```python
from build123d import *

# Parameters (mm, degrees)
F0_W     = 80
F0_H     = 40
F1_DEPTH = 5
F2_W     = 30
F2_H     = 5.5
F3_DEPTH = 20
F4_W     = 40
F4_H     = 7
F5_DEPTH = 22.4


with BuildPart() as f1:
    # F0 (on Top) → F1 (new body)
    with BuildSketch(Plane.XY):
        Rectangle(F0_W, F0_H)
    extrude(amount=F1_DEPTH)

    # F2 (on face) → F3 (join)
    with BuildSketch(Plane.XY.offset(5)):
        with Locations((-25, -17.25)):
            Rectangle(F2_W, F2_H)
        with Locations((-25, 17.25)):
            Rectangle(F2_W, F2_H)
    extrude(amount=F3_DEPTH)

    # F4 (on face) → F5 (cut)
    with BuildSketch(Plane.XY.offset(5)):
        with Locations((15, 0)):
            Rectangle(F4_W, F4_H)
    extrude(amount=-F5_DEPTH, mode=Mode.SUBTRACT)


solid = f1.part
```
The listing builds one solid part. Answer for the finished solid, in the listing's coordinates (mm). A direction names the side the tool comes from. Give positions to 0.01 mm unless a question says otherwise; leave off trailing zeros. Order: outer loops, then holes, each group sorted by start corner. A loop starts at its lowest first (then second) coordinate and runs counter-clockwise, first axis right, second up. Notation, with made-up numbers: (-39, 62) -> (18, 62) arc R27 ccw to (18, 97) -> close; hole circle Ø10 at (42.25, 34). An arc over 180 degrees is marked (long way). Answer as a JSON object with one key per item and string values. Group by question number.
Item 1: The part is cut by section D-D on x = -14.5. Write down the section's boundary in (y, z).
Item 2: Consider L1, parallel to Y at x = -30.5, z = 13.75; L2, parallel to X at y = 18, z = 5.5; L3, parallel to Z at x = 21, y = 11. Determine where each line is inside the solid, lowest interval first. Write a range as from..to.
Item 3: Flat-ended cylindrical pins translate along their axes: pin 1 (10 mm diameter, centred on x = -13, y = -12, fed in from +Z); pin 2 (20 mm diameter, centred on x = -18, y = 0, fed in from +Z); pin 3 (6 mm diameter, centred on y = 12, z = 14, fed in from +X); pin 4 (2 mm diameter, centred on x = -1, y = -1.5, fed in from -Z). Find the tip coordinate at first contact, or state that the pin passes through.
Item 4: A tool of negligible diameter and unlimited length cuts with its end or side. For faces 1 (the flat face through (15, -3.5, 3)), 2 (the flat face through (-10, 17, 15)), 3 (the flat face through (-25, 14.5, 15)), 4 (the flat face through (-25, -17, 25)), from which of +Z, -Z, +X, -X, +Y, -Y can it reach the whole face along a straight path? Write none if from no direction.
Item 5: The part is cut by section A-A on x = 4.5. Write down the section's boundary in (y, z).
Item 6: The part is cut by section C-C on z = 2.75. Write down the section's boundary in (x, y).
Item 7: The part is cut by section B-B on z = 10.5. Write down the section's boundary in (x, y).
Item 8: Determine the mould class of faces 5 (the flat face through (-40, 0, 4)), 6 (the flat face through (15, 3.5, 3)), 7 (the flat face through (-10, -17, 15)), 8 (the flat face through (-1, 5, 5)) for opening direction X: pulls with the +X half, pulls with the -X half, needs draft (parallel to the pull), parting line crosses it, or undercut.
Result set:
{
 "1": {"outline": "(-20, 0) -> (20, 0) -> (20, 25) -> (14.5, 25) -> (14.5, 5) -> (-14.5, 5) -> (-14.5, 25) -> (-20, 25) -> close"},
 "2": {"L1": "-20..-14.5, 14.5..20", "L2": "-40..-10", "L3": "0..5"},
 "3": {"pin 1": "z = 25", "pin 2": "z = 5", "pin 3": "x = -10", "pin 4": "through"},
 "4": {"face 1": "+Z, -Z", "face 2": "+Z, +X, +Y, -Y", "face 3": "+Z, +X, -X", "face 4": "+Z, +X, -X, +Y, -Y"},
 "5": {"outline": "(-20, 0) -> (-3.5, 0) -> (-3.5, 5) -> (-20, 5) -> close; (3.5, 0) -> (20, 0) -> (20, 5) -> (3.5, 5) -> close"},
 "6": {"outline": "(-40, -20) -> (40, -20) -> (40, 20) -> (-40, 20) -> close; hole (-5, -3.5) -> (35, -3.5) -> (35, 3.5) -> (-5, 3.5) -> close"},
 "7": {"outline": "(-40, -20) -> (-10, -20) -> (-10, -14.5) -> (-40, -14.5) -> close; (-40, 14.5) -> (-10, 14.5) -> (-10, 20) -> (-40, 20) -> close"},
 "8": {"face 5": "pulls with the -X half", "face 6": "undercut", "face 7": "pulls with the +X half", "face 8": "needs draft"}
}
